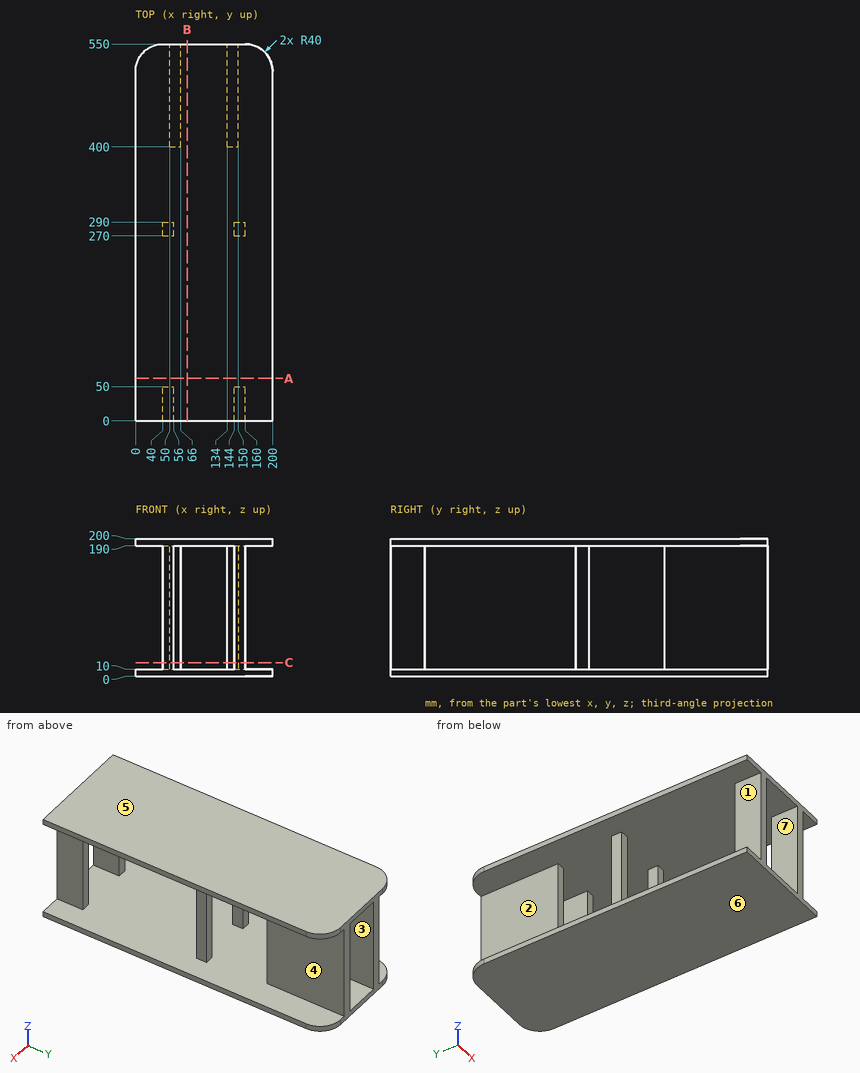
Print and shaded views of the part. All mm, measured from the part's lowest x, y and z. A direction names the side the tool comes from. Coordinates: 2 decimals unless noted, no trailing zeros. Order: outer loops, then holes, each group sorted by start corner. A loop starts at its lowest first (then second) coordinate and runs counter-clockwise, first axis right, second up. Notation, with made-up numbers: M -26,-25.5 L 12,-25.5 A20 ccw 12,-10.5 Z; hole C 79.25,-24 d6. An arc over 180 degrees is marked long. One line per question, with ' | ' between items. Start each with the question number.
Q1. Saw through at A-A (y = 62). List the corners of the cut face in (x, z).
Q2. 3-axis set-ups, long thin cutter, end or side, ignore diameter. For the marked faces 1, 2, 3 and 4: which of +Z, -Z, +X, -X, +Y, -Y reach the whole face in a straight line?
Q3. Flat gauge pins, fed straight in: pin 1 Ø22 at (y, z) = (277.5, 71) entering from -X; pin 2 Ø5 at (x, z) = (154, 132) entering from +Y; pin 3 Ø6 at (y, z) = (283.5, 71) entering from +X. Where does each tip first touch, or does it go through?
Q4. Saw through at B-B (x = 75.5). List the corners of the cut face in (y, z), then the cut area to 3 significant figures.
Q5. Saw through at C-C (z = 19.5). List the corners of the cut face in (x, y), then the cut area to 3 significant figures.
Q6. Probe L1, parallel to Z at x = 189.5, y = 133; L2, parallel to Y at x = 45.5, z = 138; L3, parallel to X at y = 480.5, z = 107.5. List the from-to ranges inside material, lowest first. Write a range as from..to.
Q7. Two-plate mould, pull along Z, no slides. Class the marked faces 5, 6 and 7: +Z half, -Z half, draft (parallel to the pull), parting line (faces both ways), or undercut.
Check values:
1) outline: M 0,0 L 200,0 L 200,10 L 0,10 Z; M 0,190 L 200,190 L 200,200 L 0,200 Z
2) face 1: -X, +Y, -Y | face 2: -X, +Y | face 3: +Y, -Y | face 4: +X, +Y
3) pin 1: stops at x = 40 | pin 2: stops at y = 290 | pin 3: stops at x = 160
4) outline: M 0,0 L 550,0 L 550,10 L 0,10 Z; M 0,190 L 550,190 L 550,200 L 0,200 Z | area: 11,000 mm2
5) outline: M 40,0 L 56,0 L 56,50 L 40,50 Z; M 40,270 L 56,270 L 56,290 L 40,290 Z; M 50,400 L 66,400 L 66,550 L 50,550 Z; M 134,400 L 150,400 L 150,550 L 134,550 Z; M 144,0 L 160,0 L 160,50 L 144,50 Z; M 144,270 L 160,270 L 160,290 L 144,290 Z | area: 7,040 mm2
6) L1: z = 0..10, 190..200 | L2: y = 0..50, 270..290 | L3: x = 50..66, 134..150
7) face 5: +Z half | face 6: -Z half | face 7: undercut
